from build123d import *

# Parameters (mm, degrees)
SKETCH_1_W          = 75
SKETCH_1_H          = 75
EXTRUDE_1_DEPTH     = 15
SKETCH_6_R          = 17.5
CUT_EXTRUDE_7_DEPTH = 1
SKETCH_7_W          = 75
SKETCH_7_H          = 75
SKETCH_7_W_2        = 55
SKETCH_7_H_2        = 55
CUT_EXTRUDE_8_DEPTH = 5
SKETCH_8_W          = 10
SKETCH_8_H          = 46
SKETCH_8_W_2        = 46
SKETCH_8_H_2        = 10
CUT_EXTRUDE_9_DEPTH = 54.967582862
SKETCH_9_W          = 85
SKETCH_9_H          = 85
SKETCH_9_W_2        = 75
SKETCH_9_H_2        = 75
EXTRUDE_2_DEPTH     = 10


with BuildPart() as part:
    # ｽｹｯﾁ1 → ﾎﾞｽ - 押し出し1 (new body)
    with BuildSketch(Plane.XY):
        Rectangle(SKETCH_1_W, SKETCH_1_H)
    extrude(amount=EXTRUDE_1_DEPTH)

    # ｽｹｯﾁ6 → ｶｯﾄ - 押し出し7 (cut)
    with BuildSketch(Plane(origin=(0, 0, 0), x_dir=(-1, 0, 0), z_dir=(0, 0, -1))):
        Circle(SKETCH_6_R)
    extrude(amount=-CUT_EXTRUDE_7_DEPTH, mode=Mode.SUBTRACT)

    # ｽｹｯﾁ7 → ｶｯﾄ - 押し出し8 (cut)
    with BuildSketch(Plane(origin=(0, 0, 0), x_dir=(-1, 0, 0), z_dir=(0, 0, -1))):
        Rectangle(SKETCH_7_W, SKETCH_7_H)
        Rectangle(SKETCH_7_W_2, SKETCH_7_H_2, mode=Mode.SUBTRACT)
    extrude(amount=-CUT_EXTRUDE_8_DEPTH, mode=Mode.SUBTRACT)

    # ｽｹｯﾁ8 → ｶｯﾄ - 押し出し9 (cut, through all)
    with BuildSketch(Plane(origin=(0, 0, 5), x_dir=(-1, 0, 0), z_dir=(0, 0, -1))):
        with Locations((-32.5, 0)):
            Rectangle(SKETCH_8_W, SKETCH_8_H)
        with Locations((32.5, 0)):
            Rectangle(SKETCH_8_W, SKETCH_8_H)
        with Locations((0, -32.5)):
            Rectangle(SKETCH_8_W_2, SKETCH_8_H_2)
        with Locations((0, 32.5)):
            Rectangle(SKETCH_8_W_2, SKETCH_8_H_2)
    extrude(amount=-CUT_EXTRUDE_9_DEPTH, mode=Mode.SUBTRACT)

    # ｽｹｯﾁ9 → ﾎﾞｽ - 押し出し2 (add)
    with BuildSketch(Plane(origin=(0, 0, 5), x_dir=(-1, 0, 0), z_dir=(0, 0, -1))):
        Rectangle(SKETCH_9_W, SKETCH_9_H)
        Rectangle(SKETCH_9_W_2, SKETCH_9_H_2, mode=Mode.SUBTRACT)
    extrude(amount=-EXTRUDE_2_DEPTH)


solid = part.part
Geometry check sheet. Reference: the model listing, model coordinates, mm. A direction names the side the tool comes from. Round coordinates to 2 decimals unless told otherwise and drop trailing zeros. Write each loop counter-clockwise with the first axis right and the second up, starting at its lowest first coordinate (ties: lowest second). Pieces come first, ordered by that corner, then holes. Notation, with made-up numbers: (72.5, 81) - (78.5, 81) arc R20 cw to (78.5, 104) - close; hole circle Ø4 at (69, -17). An arc over 180 degrees is marked (long way). One line per item, written item: value.
1. Scan lines: L1, parallel to X at y = -12, z = 11; L2, parallel to Y at x = 0, z = 0.3. Record each from-to range of solid material in increasing order.
The answers:
L1: x = -42.5 to -37.5, -27.5 to 27.5, 37.5 to 42.5
L2: y = -27.5 to -17.5, 17.5 to 27.5
2. Cross-section at C-C on y = 0. Record the boundary of the cut face in (x, z).
The answers:
outline: (-42.5, 5) - (-37.5, 5) - (-37.5, 15) - (-42.5, 15) - close; (-27.5, 0) - (-17.5, 0) - (-17.5, 1) - (17.5, 1) - (17.5, 0) - (27.5, 0) - (27.5, 15) - (-27.5, 15) - close; (37.5, 5) - (42.5, 5) - (42.5, 15) - (37.5, 15) - close
3. Depth check by flat-ended pin: pin 1 Ø10.5 at (x, y) = (6, 2.5) entering from -Z. Enter the tip coordinate at first touch or a pass-through.
The answers:
pin 1: stops at z = 1
4. Set-up check for faces 1 (the face through (0, 0, 1)), 2 (the face through (23, 32, 10)), 3 (the face through (-13, 13, 0)): record each of +Z, -Z, +X, -X, +Y, -Y from which the full face is reachable in a straight line by a thin tool's end or side.
The answers:
face 1: -Z
face 2: +Z, -Z
face 3: -Z, +X, -X, +Y, -Y
5. Mould release check, pull along X, two halves, no side actions. Record for faces 4 (the face through (1, -42.5, 10)), 5 (the face through (-42.5, -1, 10)), 6 (the face through (0, 37.5, 10)): released by +X, released by -X, zero draft, split by the parting line, or undercut.
The answers:
face 4: zero draft
face 5: released by -X
face 6: undercut
6. Cross-section at A-A on x = 34. Record the boundary of the cut face in (y, z), and give its area (3 significant figures).
The answers:
outline: (-42.5, 5) - (-23, 5) - (-23, 15) - (-42.5, 15) - close; (23, 5) - (42.5, 5) - (42.5, 15) - (23, 15) - close
area: 390 mm^2
7. Cross-section at B-B on z = 7.5. Record the boundary of the cut face in (x, y), and give its area (4 significant figures).
The answers:
outline: (-42.5, -42.5) - (42.5, -42.5) - (42.5, 42.5) - (-42.5, 42.5) - close; hole (-37.5, -23) - (-27.5, -23) - (-27.5, 23) - (-37.5, 23) - close; hole (-23, -37.5) - (23, -37.5) - (23, -27.5) - (-23, -27.5) - close; hole (-23, 27.5) - (23, 27.5) - (23, 37.5) - (-23, 37.5) - close; hole (27.5, -23) - (37.5, -23) - (37.5, 23) - (27.5, 23) - close
area: 5,385 mm^2
